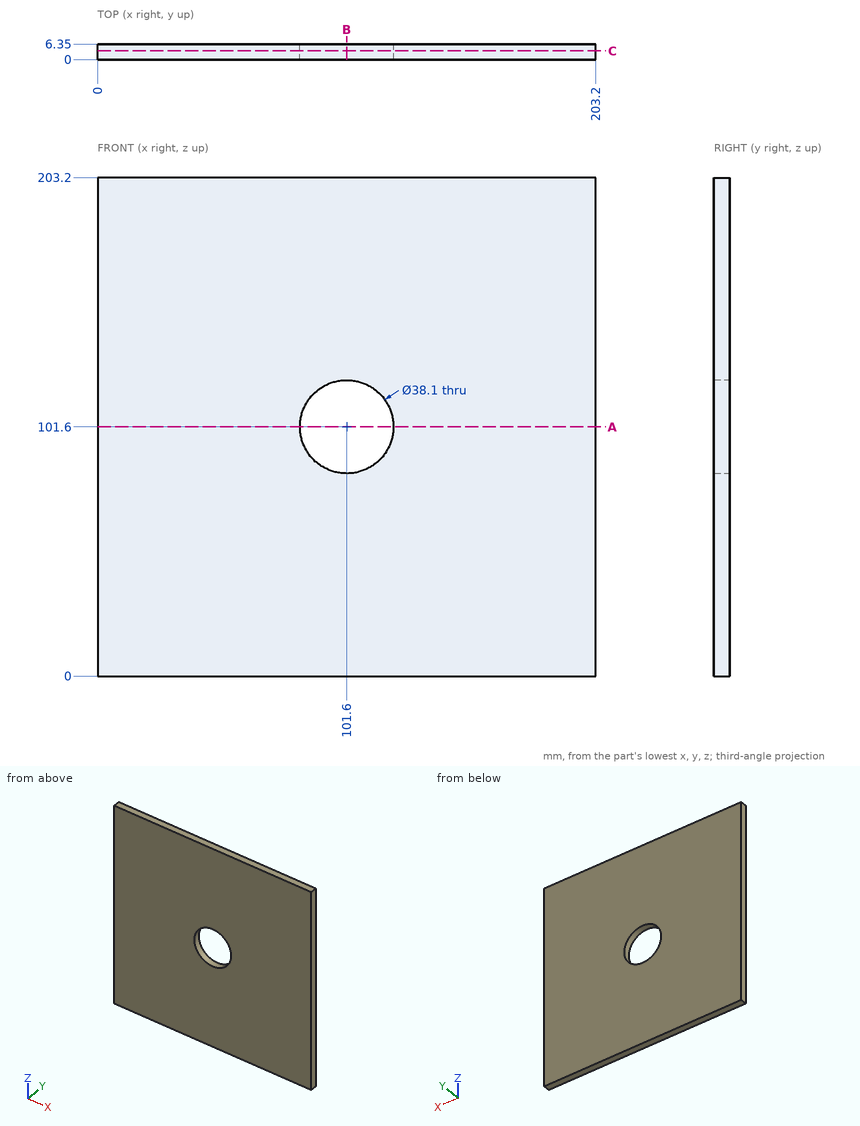
Can you work these out from the drawing? Everything is in mm from the part's minimum corner. Coordinates: 2 decimals unless noted, no trailing zeros. Write each loop counter-clockwise with the first axis right and the second up, starting at its lowest first coordinate (ties: lowest second). Pieces come first, ordered by that corner, then holes. Notation, with made-up numbers: (-2.75, 32.25) -> (3.25, 32.25) arc R12 cw to (3.25, 47.25) -> close; hole circle Ø8 at (52, -10). An arc over 180 degrees is marked (long way). Write item = value, one per line.
(1) Imagine slicing it at B-B (x = 101.6). Please give me the cut outline in (y, z).
Verdict:
outline = (0, 0) -> (6.35, 0) -> (6.35, 82.55) -> (0, 82.55) -> close; (0, 120.65) -> (6.35, 120.65) -> (6.35, 203.2) -> (0, 203.2) -> close
(2) If I drill on probe 1 along Z at (x, y) = (101.6, 1.5); probe 2 along X at (y, z) = (2.5, 97.5); probe 3 along X at (y, z) = (2.75, 88), over which ranges is the centre line in solid material (lowest first)?
Verdict:
probe_1 = 0 to 82.55, 120.65 to 203.2
probe_2 = 0 to 83, 120.2 to 203.2
probe_3 = 0 to 88.26, 114.94 to 203.2
(3) Imagine slicing it at C-C (y = 3.5). Please give me the cut outline in (x, z), and give its area (3 significant figures).
Verdict:
outline = (0, 0) -> (203.2, 0) -> (203.2, 203.2) -> (0, 203.2) -> close; hole circle Ø38.1 at (101.6, 101.6)
area = 40,200 mm^2
(4) Imagine slicing it at A-A (z = 101.6). Please give me the cut outline in (x, y).
Verdict:
outline = (0, 0) -> (82.55, 0) -> (82.55, 6.35) -> (0, 6.35) -> close; (120.65, 0) -> (203.2, 0) -> (203.2, 6.35) -> (120.65, 6.35) -> close
